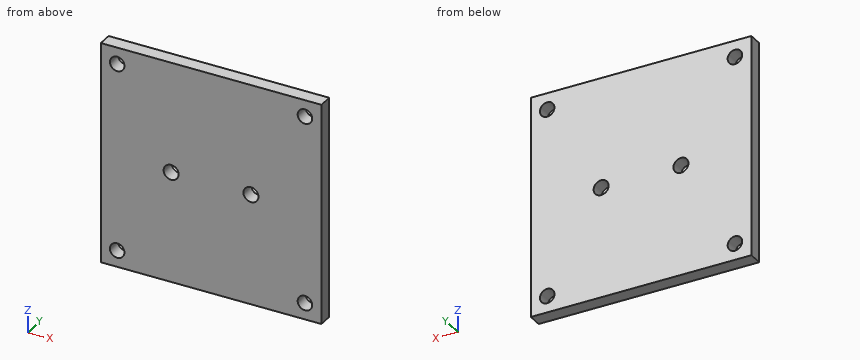
from build123d import *

# Parameters (mm, degrees)
SKETCH_1_W          = 47
SKETCH_1_H          = 47
EXTRUDE_1_DEPTH     = 3
SKETCH_3_R          = 1.55
CUT_EXTRUDE_2_DEPTH = 3
SKETCH_4_R          = 1.6
CUT_EXTRUDE_3_DEPTH = 3


with BuildPart() as part:
    # 草图1 → 凸台-拉伸1 (new body)
    with BuildSketch(Plane(origin=(0, 0, 0), x_dir=(1, 0, 0), z_dir=(0, 1, 0))):
        Rectangle(SKETCH_1_W, SKETCH_1_H)
    extrude(amount=EXTRUDE_1_DEPTH)

    # 草图3 → 切除-拉伸2 (cut)
    with BuildSketch(Plane.XZ):
        with Locations(Location((20, 20, 0), (0, 0, 270))):
            Circle(SKETCH_3_R)
        with Locations(Location((-20, 20, 0), (0, 0, 90))):
            Circle(SKETCH_3_R)
        with Locations(Location((20, -20, 0), (0, 0, 90))):
            Circle(SKETCH_3_R)
        with Locations(Location((-20, -20, 0), (0, 0, 270))):
            Circle(SKETCH_3_R)
    extrude(amount=-CUT_EXTRUDE_2_DEPTH, mode=Mode.SUBTRACT)

    # 草图4 → 切除-拉伸3 (cut)
    with BuildSketch(Plane(origin=(0, 3, 0), x_dir=(1, 0, 0), z_dir=(0, 1, 0))):
        with Locations(Location((-8.5, 0, 0), (0, 0, 270))):
            Circle(SKETCH_4_R)
        with Locations(Location((8.5, 0, 0), (0, 0, 90))):
            Circle(SKETCH_4_R)
    extrude(amount=-CUT_EXTRUDE_3_DEPTH, mode=Mode.SUBTRACT)


solid = part.part
For this review, take the finished solid that the model builds, in its own axes (mm). Give positions to 0.01 mm unless a question says otherwise; leave off trailing zeros. Loops run counter-clockwise (first coordinate to the right, second up) from the corner with the lowest first, then second, coordinate; pieces in that order, holes last.
Item 1: Take a section at A-A, the plane x = -20. State the section outline as (y, z) points.
Item 2: For line 1 along X through (y, z) = (1.6, 0); line 2 along X through (y, z) = (2.05, 20); line 3 along Z through (x, y) = (8.5, 1.65), list the stretches that pass through material, from the lowest coordinate up.
Item 3: Take a section at D-D, the plane z = -20. State the section outline as (x, y) points, and give its area (3 significant figures).
Item 4: Insertion check: pin 1 (3.5 mm diameter, centred on x = 20, z = -20, fed in from -Y). The pin has a flat end and moves straight along its axis. Give the tip position at first contact, or say it passes through.
Item 5: Take a section at B-B, the plane x = -8.5. State the section outline as (y, z) points.
Item 6: Take a section at C-C, the plane y = 0.45. State the section outline as (x, z) points.
Calculated:
1. outline: (0, -23.5) - (3, -23.5) - (3, -21.55) - (0, -21.55) - close; (0, -18.45) - (3, -18.45) - (3, 18.45) - (0, 18.45) - close; (0, 21.55) - (3, 21.55) - (3, 23.5) - (0, 23.5) - close
2. line 1: x = -23.5 to -10.1, -6.9 to 6.9, 10.1 to 23.5
2. line 2: x = -23.5 to -21.55, -18.45 to 18.45, 21.55 to 23.5
2. line 3: z = -23.5 to -1.6, 1.6 to 23.5
3. outline: (-23.5, 0) - (-21.55, 0) - (-21.55, 3) - (-23.5, 3) - close; (-18.45, 0) - (18.45, 0) - (18.45, 3) - (-18.45, 3) - close; (21.55, 0) - (23.5, 0) - (23.5, 3) - (21.55, 3) - close
3. area: 122 mm2
4. pin 1: stops at y = 0
5. outline: (0, -23.5) - (3, -23.5) - (3, -1.6) - (0, -1.6) - close; (0, 1.6) - (3, 1.6) - (3, 23.5) - (0, 23.5) - close
6. outline: (-23.5, -23.5) - (23.5, -23.5) - (23.5, 23.5) - (-23.5, 23.5) - close; hole circle Ø3.1 at (-20, -20); hole circle Ø3.1 at (-20, 20); hole circle Ø3.2 at (-8.5, 0); hole circle Ø3.2 at (8.5, 0); hole circle Ø3.1 at (20, -20); hole circle Ø3.1 at (20, 20)
